```python
from build123d import *

# Parameters (mm, degrees)
SKETCH001_R  = 2.5
PAD_DEPTH    = 10
SKETCH_R     = 1.7
POCKET_DEPTH = 12


with BuildPart() as part:
    # Sketch001 → Pad (new body)
    with BuildSketch(Plane.XY):
        with BuildLine():
            Line((0, 0), (100, 0))
            Line((100, 0), (120, 5))
            Line((120, 5), (100, 10))
            Line((100, 10), (-12.44949, 10))
            Line((-12.44949, 10), (-12.44949, 5.5))
            Line((-12.44949, 5.5), (-2.44949, 5.5))
            ThreePointArc((-2.44949, 4.5), (2.5, 5), (-2.44949, 5.5))
            Line((-2.44949, 4.5), (-12.44949, 4.5))
            Line((-12.44949, 4.5), (-12.44949, 0))
            Line((-12.44949, 0), (0, 0))
        make_face()
        with Locations((100, 5)):
            Circle(SKETCH001_R, mode=Mode.SUBTRACT)
    extrude(amount=PAD_DEPTH)

    # Sketch (on Face7 of Pad) → Pocket (cut)
    with BuildSketch(Plane(origin=(0, 10, 0), x_dir=(-1, 0, 0), z_dir=(0, 1, 0))):
        with Locations((7.5, 5)):
            Circle(SKETCH_R)
    extrude(amount=-POCKET_DEPTH, mode=Mode.SUBTRACT)


solid = part.part
```
Work out the finished part from the listing and answer in its coordinate system (mm). A direction names the side the tool comes from. Give positions to 0.01 mm unless a question says otherwise; leave off trailing zeros. Order: outer loops, then holes, each group sorted by start corner. A loop starts at its lowest first (then second) coordinate and runs counter-clockwise, first axis right, second up. Notation, with made-up numbers: (-37, 43.25) - (-14, 43.25) arc R3 cw to (-14, 48.25) - close; hole circle Ø10 at (35, 78). An arc over 180 degrees is marked (long way). One line per item, written item: value. Start each with the question number.
1. Section C-C, the plane x = 109 is taken. Write down the section's boundary in (y, z).
2. Consider line 1 (Z direction, x = -7.5, y = 7); line 2 (Y direction, x = 0, z = 3.25); line 3 (Y direction, x = 0.5, z = 6). Determine where each line is inside the solid, lowest interval first.
3. For a pull along X with two mould halves and no side action, classify faces 1 (the face through (102.385, 5.751, 4.93)), 2 (the face through (2.5, 4.9, 4.9)), 3 (the face through (109.86, 2.465, 4.93)), 4 (the face through (-8, 5.5, 3)) as released by +X, released by -X, zero draft, split by the parting line, or undercut.
4. Section B-B, the plane x = 0 is taken. Write down the section's boundary in (y, z), then the cut area to 3 significant figures.
5. Which of the six approach directions +Z, -Z, +X, -X, +Y, -Y give full straight-line access (tool end or side, diameter ignored) to faces 5 (the face through (-7, 4.5, 3)), 6 (the face through (-12.449, 2, 5))?
6. Section A-A, the plane z = 5 is taken. Write down the section's boundary in (x, y).
7. This flat-tipped pin is pushed along its axis until it touches: pin 1 Ø4.5 at (x, y) = (0, 5) entering from -Z. Where does it stop, or does it pass through?
Filled sheet:
1. outline: (2.25, 0) - (7.75, 0) - (7.75, 10) - (2.25, 10) - close
2. line 1: 0 to 3.3, 6.7 to 10
2. line 2: 0 to 2.5, 7.5 to 10
2. line 3: 0 to 2.55, 7.45 to 10
3. face 1: undercut
3. face 2: undercut
3. face 3: released by +X
3. face 4: zero draft
4. outline: (0, 0) - (2.5, 0) - (2.5, 10) - (0, 10) - close; (7.5, 0) - (10, 0) - (10, 10) - (7.5, 10) - close
4. area: 50.0 mm²
5. face 5: +Z, -Z, -X
5. face 6: +Z, -Z, -X, +Y, -Y
6. outline: (-12.45, 0) - (-9.2, 0) - (-9.2, 4.5) - (-12.45, 4.5) - close; (-12.45, 5.5) - (-9.2, 5.5) - (-9.2, 10) - (-12.45, 10) - close; (-5.8, 0) - (100, 0) - (120, 5) - (100, 10) - (-5.8, 10) - (-5.8, 5.5) - (-2.45, 5.5) arc R2.5 cw (long way) to (-2.45, 4.5) - (-5.8, 4.5) - close; hole circle Ø5 at (100, 5)
7. pin 1: through
